```python
from build123d import *

# Parameters (mm, degrees)
F1_DEPTH = 57.15
F3_D     = 11.1125
F5_D     = 11.1125
F7_D     = 25.4
F7_DEPTH = 12.7
F7_TIP   = 7.6309298617


with BuildPart() as f1:
    # F0 (on Front) → F1 (new body)
    with BuildSketch(Plane.XZ):
        Polygon((2451.1, 0), (0, 0), (0, -76.2), (38.1, -114.3), (2413, -114.3), (2451.1, -76.2), align=None)
    extrude(amount=F1_DEPTH)

    # F3 (through all)
    with Locations(Plane.XY):
        with Locations((104.775, -28.575), (822.325, -28.575), (1628.775, -28.575), (2346.325, -28.575)):
            Hole(F3_D / 2)

    # F5 (through all)
    with Locations(Plane.XZ.offset(57.15)):
        with Locations((350.8375, -57.15), (419.1, -57.15), (2032, -57.15), (2100.2625, -57.15)):
            Hole(F5_D / 2)

    # F7
    with Locations(Plane.XZ.offset(57.15)):
        with Locations((1231.9, -50.8)):
            Hole(F7_D / 2, depth=F7_DEPTH)
            with Locations((0, 0, -(F7_DEPTH + F7_TIP / 2))):  # 118° drill point
                Cone(0, F7_D / 2, F7_TIP, mode=Mode.SUBTRACT)


solid = f1.part
```
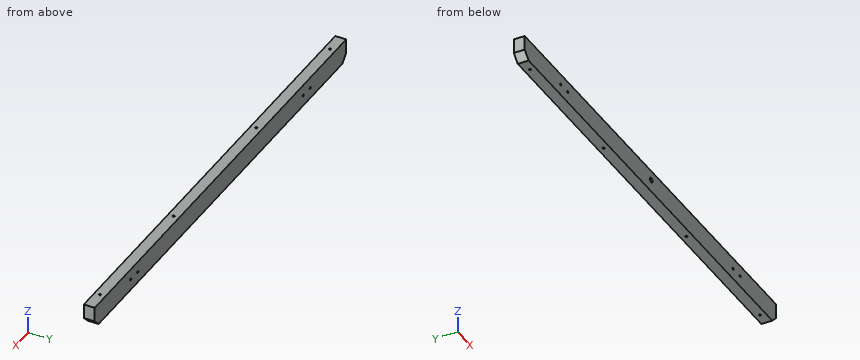
The listing builds one solid part. Answer for the finished solid, in the listing's coordinates (mm). Round coordinates to 2 decimals unless told otherwise and drop trailing zeros. Use one line per item in the form item = value.
1. Flat-ended cylindrical pins translate along their axes: pin 1 Ø3 at (y, z) = (-44, -86.5) entering from -X; pin 2 Ø9 at (x, y) = (104.775, -28.575) entering from +Z. Find the tip coordinate at first contact, or state that the pin passes through.
Answer key:
pin_1 = 8.8
pin_2 = through
2. Find the intervals of material crossed by probe 1 along X at (y, z) = (-29, -74.5); probe 2 along X at (y, z) = (-30.5, -70.5); probe 3 along Z at (x, y) = (1231.9, -51), in increasing order. Write a range as [from, to].
Answer key:
probe_1 = [0, 99.24], [110.31, 816.79], [827.86, 1623.24], [1634.31, 2340.79], [2351.86, 2451.1]
probe_2 = [0, 99.56], [109.99, 817.11], [827.54, 1623.56], [1633.99, 2341.11], [2351.54, 2451.1]
probe_3 = [-114.3, -63.5], [-38.1, 0]
3. The part is cut by section A-A on z = -94.5. Give the number of separate pieces and of enclosed holes in the cut face, and give its area (3 significant figures).
Answer key:
separate_pieces = 1
enclosed_holes = 4
area = 138,000 mm²
